from build123d import *

# Parameters (mm, degrees)
F1_DEPTH = 3
F2_R     = 0.5


# Not quite as in the source:
# - a feature names something its author has since deleted; it is built from what else it names


with BuildPart() as f1:
    # F0 (on Front) → F1 (new body)
    with BuildSketch(Plane.XZ):
        with BuildLine():
            ThreePointArc((9.9727571462, -0.7376414454), (9.9931869657, -0.3690721728), (10, 0))
            ThreePointArc((10, 0), (9.9931869657, 0.3690721728), (9.9727571462, 0.7376414454))
            ThreePointArc((9.9727571462, 0.7376414454), (9.7492791218, 2.2252093396), (9.3051943444, 3.6624251819))
            ThreePointArc((9.3051943444, 3.6624251819), (9.009688679, 4.3388373912), (8.6650930875, 4.9916091379))
            ThreePointArc((8.6650930875, 4.9916091379), (7.8183148247, 6.2348980186), (6.7946236819, 7.3371035853))
            ThreePointArc((6.7946236819, 7.3371035853), (6.2348980186, 7.8183148247), (5.6412010723, 8.2569274226))
            ThreePointArc((5.6412010723, 8.2569274226), (4.3388373912, 9.009688679), (2.9382944686, 9.5585786399))
            ThreePointArc((2.9382944686, 9.5585786399), (2.2252093396, 9.7492791218), (1.5, 9.8868599666))
            ThreePointArc((1.5, 9.8868599666), (0, 10), (-1.5, 9.8868599666))
            ThreePointArc((-1.5, 9.8868599666), (-2.2252093396, 9.7492791218), (-2.9382944686, 9.5585786399))
            ThreePointArc((-2.9382944686, 9.5585786399), (-4.3388373912, 9.009688679), (-5.6412010723, 8.2569274226))
            ThreePointArc((-5.6412010723, 8.2569274226), (-6.2348980186, 7.8183148247), (-6.7946236819, 7.3371035853))
            ThreePointArc((-6.7946236819, 7.3371035853), (-7.8183148247, 6.2348980186), (-8.6650930875, 4.9916091379))
            ThreePointArc((-8.6650930875, 4.9916091379), (-9.009688679, 4.3388373912), (-9.3051943444, 3.6624251819))
            ThreePointArc((-9.3051943444, 3.6624251819), (-9.7492791218, 2.2252093396), (-9.9727571462, 0.7376414454))
            ThreePointArc((-9.9727571462, 0.7376414454), (-10, 0), (-9.9727571462, -0.7376414454))
            ThreePointArc((-9.9727571462, -0.7376414454), (-9.7492791218, -2.2252093396), (-9.3051943444, -3.6624251819))
            ThreePointArc((-9.3051943444, -3.6624251819), (-9.009688679, -4.3388373912), (-8.6650930875, -4.9916091379))
            ThreePointArc((-8.6650930875, -4.9916091379), (-7.8183148247, -6.2348980186), (-6.7946236819, -7.3371035853))
            ThreePointArc((-6.7946236819, -7.3371035853), (-6.2348980186, -7.8183148247), (-5.6412010723, -8.2569274226))
            ThreePointArc((-5.6412010723, -8.2569274226), (-4.3388373912, -9.009688679), (-2.9382944686, -9.5585786399))
            ThreePointArc((-2.9382944686, -9.5585786399), (-2.2252093396, -9.7492791218), (-1.5, -9.8868599666))
            ThreePointArc((-1.5, -9.8868599666), (0, -10), (1.5, -9.8868599666))
            ThreePointArc((1.5, -9.8868599666), (2.2252093396, -9.7492791218), (2.9382944686, -9.5585786399))
            ThreePointArc((2.9382944686, -9.5585786399), (4.3388373912, -9.009688679), (5.6412010723, -8.2569274226))
            ThreePointArc((5.6412010723, -8.2569274226), (6.2348980186, -7.8183148247), (6.7946236819, -7.3371035853))
            ThreePointArc((6.7946236819, -7.3371035853), (7.8183148247, -6.2348980186), (8.6650930875, -4.9916091379))
            ThreePointArc((8.6650930875, -4.9916091379), (9.009688679, -4.3388373912), (9.3051943444, -3.6624251819))
            ThreePointArc((9.3051943444, -3.6624251819), (9.7492791218, -2.2252093396), (9.9727571462, -0.7376414454))
        make_face()
        with BuildLine():
            ThreePointArc((0, 1.5), (1.0606601718, 1.0606601718), (1.5, 0))
            ThreePointArc((1.5, 0), (1.0606601718, -1.0606601718), (0, -1.5))
            ThreePointArc((0, -1.5), (-1.5, 0), (0, 1.5))
        make_face(mode=Mode.SUBTRACT)
        with BuildLine():
            ThreePointArc((1.5, 6), (1.0606601718, 4.9393398282), (0, 4.5))
            ThreePointArc((0, 4.5), (-1.0606601718, 7.0606601718), (1.5, 6))
        make_face(mode=Mode.SUBTRACT)
        with BuildLine():
            ThreePointArc((-5.6412010723, 8.2569274226), (-4.3388373912, 9.009688679), (-2.9382944686, 9.5585786399))
            ThreePointArc((-2.9382944686, 9.5585786399), (-3.9281759427, 10.8096541208), (-5.1466158007, 11.8394402655))
            Line((-5.1466158007, 11.8394402655), (-6.0475846686, 11.4055565264))
            ThreePointArc((-6.0475846686, 11.4055565264), (-6.002150266, 9.8108807266), (-5.6412010723, 8.2569274226))
        make_face()
        with BuildLine():
            ThreePointArc((-1.5, 9.8868599666), (0, 10), (1.5, 9.8868599666))
            ThreePointArc((1.5, 9.8868599666), (1.1509689165, 11.4435335015), (0.5, 12.9))
            Line((0.5, 12.9), (-0.5, 12.9))
            ThreePointArc((-0.5, 12.9), (-1.1509689165, 11.4435335015), (-1.5, 9.8868599666))
        make_face()
        with BuildLine():
            ThreePointArc((-8.6650930875, 4.9916091379), (-7.8183148247, 6.2348980186), (-6.7946236819, 7.3371035853))
            ThreePointArc((-6.7946236819, 7.3371035853), (-8.2292973805, 8.0347901697), (-9.7738812229, 8.4339341852))
            Line((-9.7738812229, 8.4339341852), (-10.3973710248, 7.6521027027))
            ThreePointArc((-10.3973710248, 7.6521027027), (-9.6645321438, 6.2350627012), (-8.6650930875, 4.9916091379))
        make_face()
        with BuildLine():
            ThreePointArc((-9.9727571462, 0.7376414454), (-9.7492791218, 2.2252093396), (-9.3051943444, 3.6624251819))
            ThreePointArc((-9.3051943444, 3.6624251819), (-10.9005055464, 3.6685374852), (-12.4653096002, 3.3579840041))
            Line((-12.4653096002, 3.3579840041), (-12.6878305341, 2.3830560919))
            ThreePointArc((-12.6878305341, 2.3830560919), (-11.4127349029, 1.4243140398), (-9.9727571462, 0.7376414454))
        make_face()
        with BuildLine():
            ThreePointArc((-12.4653096002, -3.3579840041), (-10.9005055464, -3.6685374852), (-9.3051943444, -3.6624251819))
            ThreePointArc((-9.3051943444, -3.6624251819), (-9.7492791218, -2.2252093396), (-9.9727571462, -0.7376414454))
            ThreePointArc((-9.9727571462, -0.7376414454), (-11.4127349029, -1.4243140398), (-12.6878305341, -2.3830560919))
            Line((-12.6878305341, -2.3830560919), (-12.4653096002, -3.3579840041))
        make_face()
        with BuildLine():
            ThreePointArc((-9.7738812229, -8.4339341852), (-8.2292973805, -8.0347901697), (-6.7946236819, -7.3371035853))
            ThreePointArc((-6.7946236819, -7.3371035853), (-7.8183148247, -6.2348980186), (-8.6650930875, -4.9916091379))
            ThreePointArc((-8.6650930875, -4.9916091379), (-9.6645321438, -6.2350627012), (-10.3973710248, -7.6521027027))
            Line((-10.3973710248, -7.6521027027), (-9.7738812229, -8.4339341852))
        make_face()
        with BuildLine():
            ThreePointArc((-5.1466158007, -11.8394402655), (-3.9281759427, -10.8096541208), (-2.9382944686, -9.5585786399))
            ThreePointArc((-2.9382944686, -9.5585786399), (-4.3388373912, -9.009688679), (-5.6412010723, -8.2569274226))
            ThreePointArc((-5.6412010723, -8.2569274226), (-6.002150266, -9.8108807266), (-6.0475846686, -11.4055565264))
            Line((-6.0475846686, -11.4055565264), (-5.1466158007, -11.8394402655))
        make_face()
        with BuildLine():
            ThreePointArc((0.5, -12.9), (1.1509689165, -11.4435335015), (1.5, -9.8868599666))
            ThreePointArc((1.5, -9.8868599666), (0, -10), (-1.5, -9.8868599666))
            ThreePointArc((-1.5, -9.8868599666), (-1.1509689165, -11.4435335015), (-0.5, -12.9))
            Line((-0.5, -12.9), (0.5, -12.9))
        make_face()
        with BuildLine():
            ThreePointArc((6.0475846686, -11.4055565264), (6.002150266, -9.8108807266), (5.6412010723, -8.2569274226))
            ThreePointArc((5.6412010723, -8.2569274226), (4.3388373912, -9.009688679), (2.9382944686, -9.5585786399))
            ThreePointArc((2.9382944686, -9.5585786399), (3.9281759427, -10.8096541208), (5.1466158007, -11.8394402655))
            Line((5.1466158007, -11.8394402655), (6.0475846686, -11.4055565264))
        make_face()
        with BuildLine():
            ThreePointArc((10.3973710248, -7.6521027027), (9.6645321438, -6.2350627012), (8.6650930875, -4.9916091379))
            ThreePointArc((8.6650930875, -4.9916091379), (7.8183148247, -6.2348980186), (6.7946236819, -7.3371035853))
            ThreePointArc((6.7946236819, -7.3371035853), (8.2292973805, -8.0347901697), (9.7738812229, -8.4339341852))
            Line((9.7738812229, -8.4339341852), (10.3973710248, -7.6521027027))
        make_face()
        with BuildLine():
            ThreePointArc((12.6878305341, -2.3830560919), (11.4127349029, -1.4243140398), (9.9727571462, -0.7376414454))
            ThreePointArc((9.9727571462, -0.7376414454), (9.7492791218, -2.2252093396), (9.3051943444, -3.6624251819))
            ThreePointArc((9.3051943444, -3.6624251819), (10.9005055464, -3.6685374852), (12.4653096002, -3.3579840041))
            Line((12.4653096002, -3.3579840041), (12.6878305341, -2.3830560919))
        make_face()
        with BuildLine():
            ThreePointArc((9.3051943444, 3.6624251819), (9.7492791218, 2.2252093396), (9.9727571462, 0.7376414454))
            ThreePointArc((9.9727571462, 0.7376414454), (11.4127349029, 1.4243140398), (12.6878305341, 2.3830560919))
            Line((12.6878305341, 2.3830560919), (12.4653096002, 3.3579840041))
            ThreePointArc((12.4653096002, 3.3579840041), (10.9005055464, 3.6685374852), (9.3051943444, 3.6624251819))
        make_face()
        with BuildLine():
            ThreePointArc((6.7946236819, 7.3371035853), (7.8183148247, 6.2348980186), (8.6650930875, 4.9916091379))
            ThreePointArc((8.6650930875, 4.9916091379), (9.6645321438, 6.2350627012), (10.3973710248, 7.6521027027))
            Line((10.3973710248, 7.6521027027), (9.7738812229, 8.4339341852))
            ThreePointArc((9.7738812229, 8.4339341852), (8.2292973805, 8.0347901697), (6.7946236819, 7.3371035853))
        make_face()
        with BuildLine():
            ThreePointArc((2.9382944686, 9.5585786399), (4.3388373912, 9.009688679), (5.6412010723, 8.2569274226))
            ThreePointArc((5.6412010723, 8.2569274226), (6.002150266, 9.8108807266), (6.0475846686, 11.4055565264))
            Line((6.0475846686, 11.4055565264), (5.1466158007, 11.8394402655))
            ThreePointArc((5.1466158007, 11.8394402655), (3.9281759427, 10.8096541208), (2.9382944686, 9.5585786399))
        make_face()
    extrude(amount=F1_DEPTH)

    # F2
    f2_edges = [f1.edges().sort_by_distance(p)[0] for p in [
        (-5.146616, -1.5, 11.83944),
        (-6.047585, -1.5, 11.405557),
        (-9.773881, -1.5, 8.433934),
        (-10.397371, -1.5, 7.652103),
        (-0.5, -1.5, 12.9),
        (0.5, -1.5, 12.9),
        (5.146616, -1.5, 11.83944),
        (6.047585, -1.5, 11.405557),
        (9.773881, -1.5, 8.433934),
        (10.397371, -1.5, 7.652103),
        (12.46531, -1.5, 3.357984),
        (12.687831, -1.5, 2.383056),
        (12.687831, -1.5, -2.383056),
        (12.46531, -1.5, -3.357984),
        (10.397371, -1.5, -7.652103),
        (9.773881, -1.5, -8.433934),
        (6.047585, -1.5, -11.405557),
        (5.146616, -1.5, -11.83944),
        (0.5, -1.5, -12.9),
        (-0.5, -1.5, -12.9),
        (-5.146616, -1.5, -11.83944),
        (-6.047585, -1.5, -11.405557),
        (-12.46531, -1.5, 3.357984),
        (-12.687831, -1.5, 2.383056),
        (-12.687831, -1.5, -2.383056),
        (-12.46531, -1.5, -3.357984),
        (-9.773881, -1.5, -8.433934),
        (-10.397371, -1.5, -7.652103),
    ]]
    fillet(f2_edges, radius=F2_R)


solid = f1.part
The listing builds one solid part. Answer for the finished solid, in the listing's coordinates (mm). A direction names the side the tool comes from. Give positions to 0.01 mm unless a question says otherwise; leave off trailing zeros. Order: outer loops, then holes, each group sorted by start corner. A loop starts at its lowest first (then second) coordinate and runs counter-clockwise, first axis right, second up. Notation, with made-up numbers: (-1, -24.5) -> (42, -24.5) arc R22 ccw to (42, 10.5) -> close; hole circle Ø4 at (27.5, 34.5). An arc over 180 degrees is marked (long way). Put each result on its own line as item: value.
Item 1: A cutting plane is placed at D-D on x = -6.5. Give the vertices of the cut face in (y, z).
Established:
outline: (-3, -7.6) -> (0, -7.6) -> (0, 7.6) -> (-3, 7.6) -> close
Item 2: A cutting plane is placed at C-C on z = -6.5. Give the vertices of the cut face in (x, y), plus the area to 3 significant figures.
Established:
outline: (-9.83, -3) -> (9.83, -3) -> (9.83, 0) -> (-9.83, 0) -> close
area: 59.0 mm^2
Item 3: A cutting plane is placed at B-B on y = -1.5. Count the separate pieces of the cut face and the enclosed holes in it, plus the area to 3 significant figures.
Established:
separate pieces: 1
enclosed holes: 2
area: 390 mm^2
Item 4: For a pull along X with two mould halves and no side action, classify faces 1 (the face through (-9.57, -1.48, -6.09)), 2 (the face through (3.809, -1.479, -10.684)) as released by +X, released by -X, zero draft, split by the parting line, or undercut.
Established:
face 1: released by -X
face 2: undercut
Item 5: Given P1, Ø1.5, axis at y = -1.5, z = 0.5, coming from the +X side; P2, Ø1.5, axis at x = 9.5, y = -0.5, coming from the -Z side, each flat-ended and moving along its own axis, determine where each tip first touches the part or whether it passes through.
Established:
P1: stops at x = 11.11
P2: stops at z = -8.39
Item 6: For faces 3 (the face through (-1.204, -1.479, -11.279)), 4 (the face through (1.204, -1.479, 11.279)), 5 (the face through (-11.264, -1.479, -1.336)), determine the directions among +Z, -Z, +X, -X, +Y, -Y from which every point of the face is accessible in a straight line to the end or side of a thin tool.
Established:
face 3: -Z, +Y, -Y
face 4: +Z, +Y, -Y
face 5: -X, +Y, -Y
Item 7: Straight lines are drawn through the part: line 1 (X direction, y = -1.2, z = 10); line 2 (X direction, y = -2.9, z = 10.5); line 3 (Z direction, x = -9.25, y = -2.7). For each, find the intervals that lie inside material, in ascending order.
Established:
line 1: x = -6.02 to -3.24, -1.49 to 1.49, 3.24 to 6.02
line 2: x = -6.06 to -3.64, -1.4 to 1.4, 3.64 to 6.06
line 3: z = -8.34 to -5.66, -3.8 to 3.8, 5.66 to 8.34
Item 8: A cutting plane is placed at A-A on x = -11. Give the vertices of the cut face in (y, z), plus the area to 3 significant figures.
Established:
outline: (-3, -3.66) -> (0, -3.66) -> (0, -1.19) -> (-3, -1.19) -> close; (-3, 1.19) -> (0, 1.19) -> (0, 3.66) -> (-3, 3.66) -> close
area: 14.8 mm^2
